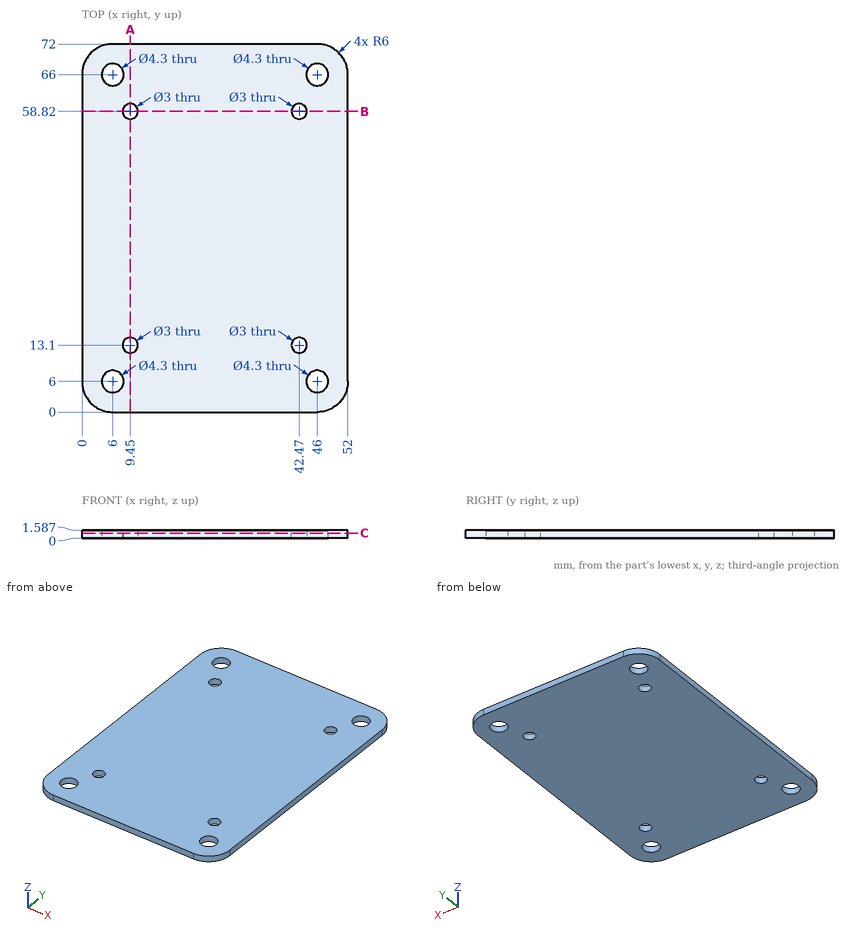
Study the drawing (mm; zero at the part's minimum x, y, z) and answer. Give positions to 0.01 mm unless a question says otherwise; leave off trailing zeros. Write each loop counter-clockwise with the first axis right and the second up, starting at its lowest first coordinate (ties: lowest second). Pieces come first, ordered by that corner, then holes. Notation, with made-up numbers: (-30.75, 30.25) - (14.25, 30.25) arc R30 ccw to (14.25, 59.25) - close; hole circle Ø6 at (16, 8.25). An arc over 180 degrees is marked (long way). One line per question, with ' | ' between items. Start each with the question number.
1. Section A-A, the plane x = 9.45 is taken. Determine the outline of the cut face in (y, z), then the cut area to 3 significant figures.
2. Given P1, Ø2.5, axis at x = 42.47, y = 13.1, coming from the +Z side, flat-ended and moving along its own axis, determine where the tip first touches the part or whether it passes through.
3. Section C-C, the plane z = 1 is taken. Count the separate pieces of the cut face and the enclosed holes in it, then the cut area to 3 significant figures.
4. Straight lines are drawn through the part: line 1 (Y direction, x = 6, z = 0.75); line 2 (Y direction, x = 9.45, z = 0.3); line 3 (X direction, y = 66.5, z = 1.3). For each, find the intervals that lie inside material, in ascending order.
5. Section B-B, the plane y = 58.82 is taken. Determine the outline of the cut face in (x, z).
Result:
1) outline: (0, 0) - (11.6, 0) - (11.6, 1.59) - (0, 1.59) - close; (14.6, 0) - (57.32, 0) - (57.32, 1.59) - (14.6, 1.59) - close; (60.32, 0) - (72, 0) - (72, 1.59) - (60.32, 1.59) - close | area: 105 mm2
2) P1: passes through
3) separate pieces: 1 | enclosed holes: 8 | area: 3,630 mm2
4) line 1: y = 0 to 3.85, 8.15 to 63.85, 68.15 to 72 | line 2: y = 0 to 11.6, 14.6 to 57.32, 60.32 to 72 | line 3: x = 0.02 to 3.91, 8.09 to 43.91, 48.09 to 51.98
5) outline: (0, 0) - (7.95, 0) - (7.95, 1.59) - (0, 1.59) - close; (10.95, 0) - (40.97, 0) - (40.97, 1.59) - (10.95, 1.59) - close; (43.97, 0) - (52, 0) - (52, 1.59) - (43.97, 1.59) - close
